Input: part model. Units: mm. Frame: model coordinates. Face numbers are marked on the shaded views. A direction names the side the tool comes from. Give positions to 0.01 mm unless a question says otherwise; leave off trailing zeros. Loops run counter-clockwise (first coordinate to the right, second up) from the corner with the lowest first, then second, coordinate; pieces in that order, holes last. Notation, with made-up numbers: (41.25, 8.5) - (67.25, 8.5) arc R21 ccw to (67.25, 30.5) - close; hole circle Ø8 at (87, -29.5). An arc over 180 degrees is marked (long way). Answer as a JSON object with one key per item and string values.
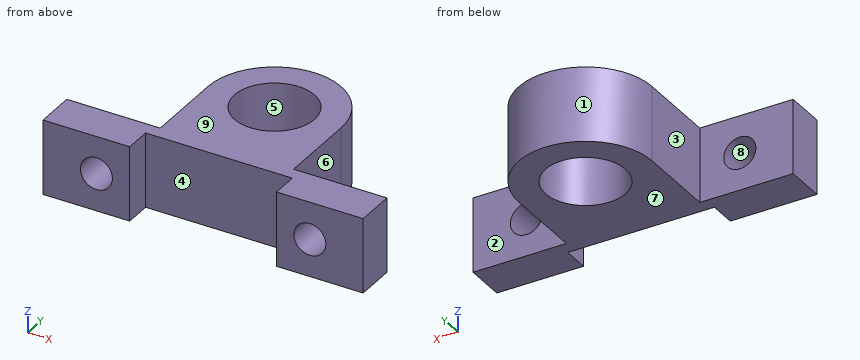
from build123d import *

# Parameters (mm, degrees)
SKETCH2_R           = 19.05
BOSS_EXTRUDE1_DEPTH = 17.78
SKETCH3_R           = 7.62
CUT_EXTRUDE1_DEPTH  = 105.888468861


with BuildPart() as part:
    # Sketch2 → Boss-Extrude1 (new, symmetric)
    with BuildSketch(Plane.XY):
        with BuildLine():
            Line((34.925, 0), (76.2, 0))
            Line((76.2, 0), (76.2, 19.05))
            Line((76.2, 19.05), (31.75, 19.05))
            Line((31.75, 19.05), (31.75, 57.15))
            ThreePointArc((31.75, 57.15), (0, 88.9), (-31.75, 57.15))
            Line((-31.75, 57.15), (-31.75, 19.05))
            Line((-31.75, 19.05), (-76.2, 19.05))
            Line((-76.2, 19.05), (-76.2, 0))
            Line((-76.2, 0), (-34.925, 0))
            Line((-34.925, 0), (-34.925, 12.7))
            Line((-34.925, 12.7), (34.925, 12.7))
            Line((34.925, 12.7), (34.925, 0))
        make_face()
        with Locations(Location((0, 57.15, 0), (0, 0, 180))):
            Circle(SKETCH2_R, mode=Mode.SUBTRACT)
    extrude(amount=BOSS_EXTRUDE1_DEPTH, both=True)

    # Sketch3 → Cut-Extrude1 (cut, through all)
    with BuildSketch(Plane(origin=(0, 19.05, 0), x_dir=(1, 0, 0), z_dir=(0, 1, 0))):
        with Locations(Location((-50.8, 0, 0), (0, 0, 180))):
            Circle(SKETCH3_R)
        with Locations(Location((50.8, 0, 0), (0, 0, 180))):
            Circle(SKETCH3_R)
    extrude(amount=-CUT_EXTRUDE1_DEPTH, mode=Mode.SUBTRACT)


solid = part.part
Item 1: Cut plane B-B (y = 7). Return loops of the section in (x, z) (3 decimals), then the cut area to 3 significant figures.
Geometry check:
{"outline": "(-76.2, -17.78) - (-34.925, -17.78) - (-34.925, 17.78) - (-76.2, 17.78) - close; (34.925, -17.78) - (76.2, -17.78) - (76.2, 17.78) - (34.925, 17.78) - close; hole circle Ø15.24 at (-50.8, 0); hole circle Ø15.24 at (50.8, 0)", "area": "2,570 mm2"}
Item 2: Mould query, pull axis Z, two halves, no side actions, for the marked faces 6, 7, 8 and 9. Classes: released by +Z, released by -Z, zero draft, split by the parting line, or undercut.
Geometry check:
{"face 6": "zero draft", "face 7": "released by -Z", "face 8": "undercut", "face 9": "released by +Z"}
Item 3: Material intervals for line 1 (Z direction, x = -50.8, y = 10); line 2 (Y direction, x = 0, z = -0.5); line 3 (X direction, y = 57, z = -2), sorted ascending. Write a range as [from, to].
Geometry check:
{"line 1": "z = [-17.78, -7.62], [7.62, 17.78]", "line 2": "y = [12.7, 38.1], [76.2, 88.9]", "line 3": "x = [-31.75, -19.05], [19.05, 31.75]"}
Item 4: Cut plane A-A (z = 0). Return loops of the section in (x, y) (3 decimals).
Geometry check:
{"outline": "(-76.2, 0) - (-58.42, 0) - (-58.42, 19.05) - (-76.2, 19.05) - close; (-43.18, 0) - (-34.925, 0) - (-34.925, 12.7) - (34.925, 12.7) - (34.925, 0) - (43.18, 0) - (43.18, 19.05) - (31.75, 19.05) - (31.75, 57.15) arc R31.75 ccw to (-31.75, 57.15) - (-31.75, 19.05) - (-43.18, 19.05) - close; (58.42, 0) - (76.2, 0) - (76.2, 19.05) - (58.42, 19.05) - close; hole circle Ø38.1 at (0, 57.15)"}
Item 5: Contact query for flat-ended pins moving along their axis: P1, Ø3, axis at x = 16.5, z = 1.5, coming from the -Y side; P2, Ø8, axis at y = 25.5, z = 6, coming from the +X side; P3, Ø12, axis at x = -9, z = 2.5, coming from the +Y side. Output: stop coordinate, or through.
Geometry check:
{"P1": "stops at y = 12.7", "P2": "stops at x = 31.75", "P3": "stops at y = 88.76"}
Item 6: Cut plane C-C (x = 50.8). Return loops of the section in (y, z).
Geometry check:
{"outline": "(0, -17.78) - (19.05, -17.78) - (19.05, -7.62) - (0, -7.62) - close; (0, 7.62) - (19.05, 7.62) - (19.05, 17.78) - (0, 17.78) - close"}
Item 7: Access query for the marked faces 1, 2, 3, 4 and 5. Directions: +Z, -Z, +X, -X, +Y, -Y. A direction counts if a zero-diameter tool reaches every point of the face in a straight line with its end or side. Return the directions, or none.
Geometry check:
{"face 1": "+Z, -Z, +Y", "face 2": "+Z, -Z, +X, +Y", "face 3": "+Z, -Z, -X, +Y", "face 4": "+Z, -Z, -Y", "face 5": "+Z, -Z"}
Item 8: Cut plane D-D (y = 17.5). Return loops of the section in (x, z).
Geometry check:
{"outline": "(-76.2, -17.78) - (76.2, -17.78) - (76.2, 17.78) - (-76.2, 17.78) - close; hole circle Ø15.24 at (-50.8, 0); hole circle Ø15.24 at (50.8, 0)"}
